Work out the finished part from the listing and answer in its coordinate system (mm). A direction names the side the tool comes from. Round coordinates to 2 decimals unless told otherwise and drop trailing zeros. Order: outer loops, then holes, each group sorted by start corner. A loop starts at its lowest first (then second) coordinate and runs counter-clockwise, first axis right, second up.
from build123d import *

# Parameters (mm, degrees)
SKETCH1_R           = 21
BOSS_EXTRUDE1_DEPTH = 2
SKETCH2_R           = 21
SKETCH2_R_2         = 3
BOSS_EXTRUDE2_DEPTH = 4
CUT_EXTRUDE1_START  = -2
SKETCH3_R           = 2
CUT_EXTRUDE1_DEPTH  = 2


with BuildPart() as part:
    # Sketch1 → Boss-Extrude1 (new body)
    with BuildSketch(Plane(origin=(0, 0, 0), x_dir=(1, 0, 0), z_dir=(0, 1, 0))):
        with Locations(Location((0, 0, 0), (0, 0, 270))):
            Circle(SKETCH1_R)
    extrude(amount=BOSS_EXTRUDE1_DEPTH)

    # Sketch2 → Boss-Extrude2 (add)
    with BuildSketch(Plane(origin=(0, 2, 0), x_dir=(1, 0, 0), z_dir=(0, 1, 0))):
        with Locations(Location((0, 0, 0), (0, 0, 270))):
            Circle(SKETCH2_R)
        with Locations(Location((0, 17, 0), (0, 0, 270))):
            Circle(SKETCH2_R_2, mode=Mode.SUBTRACT)
        with Locations(Location((14.722431864, -8.5, 0), (0, 0, 270))):
            Circle(SKETCH2_R_2, mode=Mode.SUBTRACT)
        with Locations(Location((-14.722431864, -8.5, 0), (0, 0, 270))):
            Circle(SKETCH2_R_2, mode=Mode.SUBTRACT)
        with BuildLine():
            Line((-11.5, -4.021071935), (-11.5, 9.5))
            ThreePointArc((-11.5, 9.5), (-10.914213562, 10.914213562), (-9.5, 11.5))
            Line((-9.5, 11.5), (9.5, 11.5))
            ThreePointArc((9.5, 11.5), (10.914213562, 10.914213562), (11.5, 9.5))
            Line((11.5, 9.5), (11.5, -4.021071935))
            ThreePointArc((11.5, -4.021071935), (11.972973612, -4.870920855), (12.944486373, -4.916857548))
            ThreePointArc((12.944486373, -4.916857548), (14.965992077, -4.507422083), (16.922739342, -5.159543893))
            ThreePointArc((16.922739342, -5.159543893), (17.83709693, -5.255719057), (18.443528223, -4.564675969))
            ThreePointArc((18.443528223, -4.564675969), (16.454482672, 9.5), (5.268638762, 18.254901961))
            ThreePointArc((5.268638762, 18.254901961), (4.366962246, 18.075238599), (3.993073588, 17.235294118))
            ThreePointArc((3.993073588, 17.235294118), (2.9104275, 14.256022638), (0, 13))
            ThreePointArc((0, 13), (-2.9104275, 14.256022638), (-3.993073588, 17.235294118))
            ThreePointArc((-3.993073588, 17.235294118), (-4.366962246, 18.075238599), (-5.268638762, 18.254901961))
            ThreePointArc((-5.268638762, 18.254901961), (-16.454482672, 9.5), (-18.443528223, -4.564675969))
            ThreePointArc((-18.443528223, -4.564675969), (-17.83709693, -5.255719057), (-16.922739342, -5.159543893))
            ThreePointArc((-16.922739342, -5.159543893), (-14.965992077, -4.507422083), (-12.944486373, -4.916857548))
            ThreePointArc((-12.944486373, -4.916857548), (-11.972973612, -4.870920855), (-11.5, -4.021071935))
        make_face(mode=Mode.SUBTRACT)
        with BuildLine():
            Line((9, -10.5), (-9, -10.5))
            ThreePointArc((-9, -10.5), (-10.060660172, -10.060660172), (-10.5, -9))
            Line((-10.5, -9), (-10.5, 9))
            ThreePointArc((-10.5, 9), (-10.060660172, 10.060660172), (-9, 10.5))
            Line((-9, 10.5), (9, 10.5))
            ThreePointArc((9, 10.5), (10.060660172, 10.060660172), (10.5, 9))
            Line((10.5, 9), (10.5, -9))
            ThreePointArc((10.5, -9), (10.060660172, -10.060660172), (9, -10.5))
        make_face(mode=Mode.SUBTRACT)
        with BuildLine():
            Line((11.5, -11.5), (-11.5, -11.5))
            Line((-11.5, -11.5), (-11.722431864, -11.5))
            ThreePointArc((-11.722431864, -11.5), (-12.03865963, -11.551316702), (-12.322431864, -11.7))
            ThreePointArc((-12.322431864, -11.7), (-12.617647084, -11.901452782), (-12.929665754, -12.075750225))
            ThreePointArc((-12.929665754, -12.075750225), (-13.470134683, -12.819519543), (-13.174889461, -13.690225991))
            ThreePointArc((-13.174889461, -13.690225991), (0, -19), (13.174889461, -13.690225991))
            ThreePointArc((13.174889461, -13.690225991), (13.470134683, -12.819519543), (12.929665754, -12.075750225))
            ThreePointArc((12.929665754, -12.075750225), (12.617647084, -11.901452782), (12.322431864, -11.7))
            ThreePointArc((12.322431864, -11.7), (12.03865963, -11.551316702), (11.722431864, -11.5))
            Line((11.722431864, -11.5), (11.5, -11.5))
        make_face(mode=Mode.SUBTRACT)
    extrude(amount=BOSS_EXTRUDE2_DEPTH)

    # Sketch3 → Cut-Extrude1 (cut)
    with BuildSketch(Plane(origin=(0, 2, 0), x_dir=(1, 0, 0), z_dir=(0, 1, 0)).offset(CUT_EXTRUDE1_START)):
        with Locations(Location((0, 17, 0), (0, 0, 270))):
            Circle(SKETCH3_R)
        with Locations(Location((14.722431864, -8.5, 0), (0, 0, 270))):
            Circle(SKETCH3_R)
        with Locations(Location((-14.722431864, -8.5, 0), (0, 0, 270))):
            Circle(SKETCH3_R)
        with BuildLine():
            Line((9, 7), (-9, 7))
            ThreePointArc((-9, 7), (-10.060660172, 7.439339828), (-10.5, 8.5))
            Line((-10.5, 8.5), (-10.5, 9))
            ThreePointArc((-10.5, 9), (-10.060660172, 10.060660172), (-9, 10.5))
            Line((-9, 10.5), (9, 10.5))
            ThreePointArc((9, 10.5), (10.060660172, 10.060660172), (10.5, 9))
            Line((10.5, 9), (10.5, 8.5))
            ThreePointArc((10.5, 8.5), (10.060660172, 7.439339828), (9, 7))
        make_face()
    extrude(amount=CUT_EXTRUDE1_DEPTH, mode=Mode.SUBTRACT)


solid = part.part
Item 1: Find the intervals of material crossed by line 1 along Z through (x, y) = (-8, 2.8); line 2 along X through (y, z) = (2.25, -17.5); line 3 along Z through (x, y) = (-0.5, 0.7), in increasing order.
Item 2: Given pin 1 (3 mm diameter, centred on x = 6.5, z = 3.5, fed in from +Y); pin 2 (1.2 mm diameter, centred on y = 3.5, z = -5, fed in from +X); pin 3 (1.8 mm diameter, centred on y = 3.5, z = 4.5, fed in from +X), each flat-ended and moving along its own axis, determine where each tip first touches the part or whether it passes through.
Item 3: Find section D-D (y = 3.85). State how many separate pieces and enclosed holes the cut face has, plus the area to 3 significant figures.
Item 4: For a pull along Z with two mould halves and no side action, classify faces 1 (the face through (11, 6, 3)), 2 (the face through (0, 4, 11.5)) as released by +Z, released by -Z, zero draft, split by the parting line, or undercut.
Item 5: Find section A-A (z = 8.5). Write down the section's boundary in (x, y).
Item 6: Find section C-C (x = -1.5). Write down the section's boundary in (y, z).
Item 7: A tool of negligible diameter and unlimited length cuts with its end or side. For faces 3 (the face through (-13.47, 3.97, 12.81)), 4 (the face through (-10.05, 0.99, -7.43)), from which of +Z, -Z, +X, -X, +Y, -Y can it reach the whole face along a straight path? Write none if from no direction.
Item 8: Find section B-B (z = 0). Write down the section's boundary in (x, y).
Model answer:
1. line 1: z = -19.42 to -17.23, -11.5 to -10.5, 10.5 to 11.5, 17.23 to 19.42
1. line 2: x = -11.61 to -7.4, -4.01 to -2.96, 2.96 to 4.01, 7.4 to 11.61
1. line 3: z = -20.99 to -18.94, -15.06 to -10.5, -7 to 20.99
2. pin 1: stops at y = 2
2. pin 2: stops at x = 20.53
2. pin 3: stops at x = 20.69
3. separate pieces: 1
3. enclosed holes: 6
3. area: 374 mm2
4. face 1: zero draft
4. face 2: undercut
5. outline: (-19.2, 0) - (-16.72, 0) - (-16.72, 2) - (-17.72, 2) - (-17.72, 6) - (-19.2, 6) - close; (-12.72, 0) - (12.72, 0) - (12.72, 2) - (11.72, 2) - (11.72, 6) - (10.5, 6) - (10.5, 2) - (-10.5, 2) - (-10.5, 6) - (-11.72, 6) - (-11.72, 2) - (-12.72, 2) - close; (16.72, 0) - (19.2, 0) - (19.2, 6) - (17.72, 6) - (17.72, 2) - (16.72, 2) - close
6. outline: (0, -20.95) - (6, -20.95) - (6, -19.6) - (2, -19.6) - (2, -18.32) - (0, -18.32) - close; (0, -15.68) - (2, -15.68) - (2, -14.4) - (6, -14.4) - (6, -13.29) - (2, -13.29) - (2, -11.5) - (6, -11.5) - (6, -10.5) - (0, -10.5) - close; (0, -7) - (2, -7) - (2, 10.5) - (6, 10.5) - (6, 11.5) - (2, 11.5) - (2, 18.94) - (6, 18.94) - (6, 20.95) - (0, 20.95) - close
7. face 3: +Y
7. face 4: +Y, -Y
8. outline: (-21, 0) - (21, 0) - (21, 6) - (19, 6) - (19, 2) - (11.5, 2) - (11.5, 6) - (10.5, 6) - (10.5, 2) - (-10.5, 2) - (-10.5, 6) - (-11.5, 6) - (-11.5, 2) - (-19, 2) - (-19, 6) - (-21, 6) - close
